For this review, take the finished solid that the model builds, in its own axes (mm). Face numbers are marked on the shaded views. A direction names the side the tool comes from. Coordinates: 2 decimals unless noted, no trailing zeros. Loops run counter-clockwise (first coordinate to the right, second up) from the corner with the lowest first, then second, coordinate; pieces in that order, holes last.
1. Take a section at C-C, the plane z = 6.5. State the section outline as (x, y) points, then the cut area to 3 significant figures.
2. Machinability: for the marked faces 1 and 2, which of the approach directions +Z, -Z, +X, -X, +Y, -Y give a long, thin tool a straight path to every point of the face, cutting with its end or side? Answer none if there is none.
3. To check wall thickness, follow probe 1 along X at (y, z) = (0.75, 12.25); probe 2 along Z at (x, y) = (11, 3.5); probe 3 along Y at (x, z) = (-7, 9.75). State the ranges of each line that lie inside material, in increasing order.
4. Take a section at D-D, the plane z = 1.75. State the section outline as (x, y) points.
5. Clearance check with flat-ended pins moving along their axes: P1, Ø5, axis at x = -2.5, z = 7.5, coming from the -Y side; P2, Ø0.8, axis at x = -22, y = 5.5, coming from the +Z side; P3, Ø1.1, axis at y = 5.5, z = 6, coming from the +X side. State where each tip first meets the part, or that it passes through.
6. Mouldability with a two-part tool opening along X and no side actions: class the marked faces 3, 4 and 5 as pulls with the +X half, pulls with the -X half, needs draft (parallel to the pull), parting line crosses it, or undercut.
7. Take a section at A-A, the plane y = 3.5. State the section outline as (x, z) points.
8. Take a section at B-B, the plane x = -7. State the section outline as (y, z) points, then the cut area to 3 significant figures.
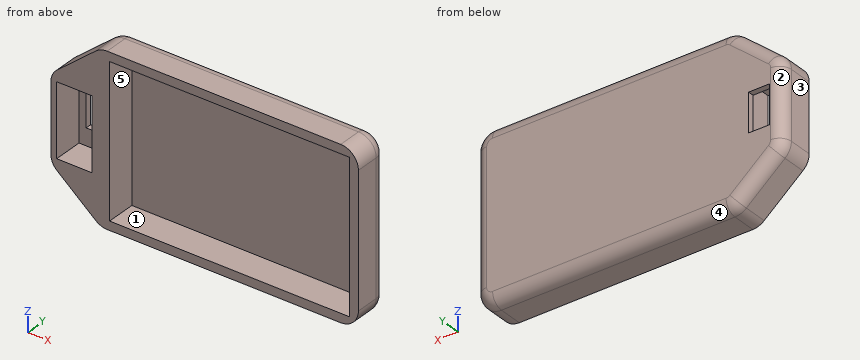
```python
from build123d import *

# Parameters (mm, degrees)
BOSS_EXTRUDE1_DEPTH = 6
SKETCH2_W           = 40.6
SKETCH2_H           = 25.4
SKETCH2_W_2         = 5.95
SKETCH2_H_2         = 12.25
CUT_EXTRUDE1_DEPTH  = 5
SKETCH4_W           = 3.5
SKETCH4_H           = 6.5
CUT_EXTRUDE2_DEPTH  = 35.473394043
FILLET1_R           = 2


with BuildPart() as part:
    # Sketch1 → Boss-Extrude1 (new body)
    with BuildSketch(Plane(origin=(0, 0, 0), x_dir=(1, 0, 0), z_dir=(0, 1, 0))):
        with BuildLine():
            Line((26.775527572, -17.868301802), (26.775527572, 4.531698198))
            ThreePointArc((26.775527572, 4.531698198), (25.896847915, 6.653018542), (23.775527572, 7.531698198))
            Line((23.775527572, 7.531698198), (-15.734378779, 7.531698198))
            ThreePointArc((-15.734378779, 7.531698198), (-16.758931033, 7.351324535), (-17.660281792, 6.831893316))
            Line((-17.660281792, 6.831893316), (-24.200375442, 1.356016089))
            ThreePointArc((-24.200375442, 1.356016089), (-24.992717178, 0.325130027), (-25.274472428, -0.944179029))
            Line((-25.274472428, -0.944179029), (-25.274472428, -12.392424575))
            ThreePointArc((-25.274472428, -12.392424575), (-24.992717178, -13.661733631), (-24.200375442, -14.692619693))
            Line((-24.200375442, -14.692619693), (-17.660281792, -20.16849692))
            ThreePointArc((-17.660281792, -20.16849692), (-16.758931033, -20.687928139), (-15.734378779, -20.868301802))
            Line((-15.734378779, -20.868301802), (23.775527572, -20.868301802))
            ThreePointArc((23.775527572, -20.868301802), (25.896847915, -19.989622146), (26.775527572, -17.868301802))
        make_face()
    extrude(amount=BOSS_EXTRUDE1_DEPTH)

    # Sketch2 → Cut-Extrude1 (cut)
    with BuildSketch(Plane(origin=(0, 0, 0), x_dir=(1, 0, 0), z_dir=(0, 1, 0))):
        with Locations((4.975527572, -6.668301802)):
            Rectangle(SKETCH2_W, SKETCH2_H)
        with Locations((-21.299472428, -6.668301802)):
            Rectangle(SKETCH2_W_2, SKETCH2_H_2)
    extrude(amount=CUT_EXTRUDE1_DEPTH, mode=Mode.SUBTRACT)

    # Sketch4 → Cut-Extrude2 (cut, through all)
    with BuildSketch(Plane(origin=(0, 6, 0), x_dir=(1, 0, 0), z_dir=(0, 1, 0))):
        with Locations((-21.299472428, -6.668301802)):
            Rectangle(SKETCH4_W, SKETCH4_H)
    extrude(amount=-CUT_EXTRUDE2_DEPTH, mode=Mode.SUBTRACT)

    # Fillet1
    fillet1_edges = [part.edges().sort_by_distance(p)[0] for p in [
        (25.896847915, 6, -6.653018542),
        (4.020574397, 6, -7.531698198),
        (-16.758931033, 6, -7.351324535),
        (-20.930328617, 6, -4.093954703),
        (-24.992717178, 6, -0.325130027),
        (-25.274472428, 6, 6.668301802),
        (-24.992717178, 6, 13.661733631),
        (-20.930328617, 6, 17.430558307),
        (-16.758931033, 6, 20.687928139),
        (4.020574397, 6, 20.868301802),
        (25.896847915, 6, 19.989622146),
        (26.775527572, 6, 6.668301802),
    ]]
    fillet(fillet1_edges, radius=FILLET1_R)


solid = part.part
```
Results list:
1. outline: (-25.27, 0) - (-24.27, 0) - (-24.27, 5) - (-23.05, 5) - (-23.05, 6) - (-23.27, 6) arc R2 ccw to (-25.27, 4) - close; (-19.55, 5) - (-18.32, 5) - (-18.32, 0) - (-15.32, 0) - (-15.32, 5) - (25.28, 5) - (25.28, 0) - (26.78, 0) - (26.78, 4) arc R2 ccw to (24.78, 6) - (-19.55, 6) - close
1. area: 74.3 mm2
2. face 1: -Y
2. face 2: +Z, -Z, -X, +Y
3. probe 1: x = -25.27 to -24.27, -18.32 to -15.32, 25.28 to 26.78
3. probe 2: z = -7.53 to -6.03, 19.37 to 20.87
3. probe 3: y = 5 to 6
4. outline: (-25.27, 0) - (-24.27, 0) - (-24.27, 5) - (-18.32, 5) - (-18.32, 0) - (-15.32, 0) - (-15.32, 5) - (25.28, 5) - (25.28, 0) - (26.78, 0) - (26.78, 4) arc R2 ccw to (24.78, 6) - (-23.27, 6) arc R2 ccw to (-25.27, 4) - close
5. P1: stops at y = 5
5. P2: stops at z = 16.23
5. P3: stops at x = 26.54
6. face 3: pulls with the -X half
6. face 4: needs draft
6. face 5: undercut
7. outline: (-25.27, 0.94) arc R3 ccw to (-24.2, -1.36) - (-17.66, -6.83) arc R3 ccw to (-15.73, -7.53) - (23.78, -7.53) arc R3 ccw to (26.78, -4.53) - (26.78, 17.87) arc R3 ccw to (23.78, 20.87) - (-15.73, 20.87) arc R3 ccw to (-17.66, 20.17) - (-24.2, 14.69) arc R3 ccw to (-25.27, 12.39) - close; hole (-24.27, 0.54) - (-18.32, 0.54) - (-18.32, 12.79) - (-24.27, 12.79) - close; hole (-15.32, -6.03) - (25.28, -6.03) - (25.28, 19.37) - (-15.32, 19.37) - close
8. outline: (0, -7.53) - (4, -7.53) arc R2 ccw to (6, -5.53) - (6, 18.87) arc R2 ccw to (4, 20.87) - (0, 20.87) - (0, 19.37) - (5, 19.37) - (5, -6.03) - (0, -6.03) - close
8. area: 41.7 mm2
